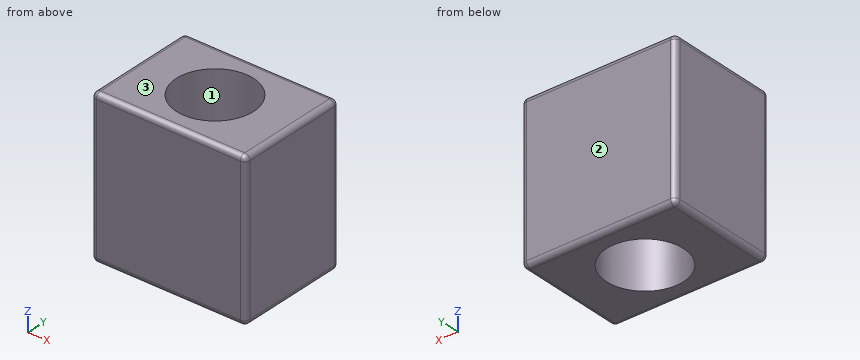
from build123d import *

# Parameters (mm, degrees)
SKETCH1_W           = 15
SKETCH1_H           = 11
SKETCH1_R           = 3.75
BOSS_EXTRUDE1_DEPTH = 7.5
FILLET1_R           = 0.5


with BuildPart() as part:
    # Sketch1 → Boss-Extrude1 (new, symmetric)
    with BuildSketch(Plane.XY):
        Rectangle(SKETCH1_W, SKETCH1_H)
        Circle(SKETCH1_R, mode=Mode.SUBTRACT)
    extrude(amount=BOSS_EXTRUDE1_DEPTH, both=True)

    # Fillet1
    fillet1_edges = [part.edges().sort_by_distance(p)[0] for p in [
        (7.5, 0, 7.5),
        (0, 5.5, 7.5),
        (-7.5, 0, 7.5),
        (0, 5.5, -7.5),
        (7.5, 0, -7.5),
        (0, -5.5, -7.5),
        (-7.5, 0, -7.5),
        (0, -5.5, 7.5),
        (-7.5, 5.5, 0),
        (7.5, 5.5, 0),
        (7.5, -5.5, 0),
        (-7.5, -5.5, 0),
    ]]
    fillet(fillet1_edges, radius=FILLET1_R)


solid = part.part
Read the model definition and answer for the solid it produces. Units are mm, in the model's axes. Face numbers are marked on the shaded views. Round coordinates to 2 decimals unless told otherwise and drop trailing zeros. Write each loop counter-clockwise with the first axis right and the second up, starting at its lowest first coordinate (ties: lowest second). Pieces come first, ordered by that corner, then holes. Notation, with made-up numbers: (13.5, -30) - (43.5, -30) arc R6 ccw to (43.5, -25) - close; hole circle Ø1 at (-20.5, 68.5). An arc over 180 degrees is marked (long way). Use a Markdown table: item, result.
(1) The part is cut by section C-C (y = 0). Write down the section's boundary in (x, z), then the cut area to 3 significant figures.
Reported:
| item | result |
|---|---|
| outline | (-7.5, -7) arc R0.5 ccw to (-7, -7.5) - (-3.75, -7.5) - (-3.75, 7.5) - (-7, 7.5) arc R0.5 ccw to (-7.5, 7) - close; (3.75, -7.5) - (7, -7.5) arc R0.5 ccw to (7.5, -7) - (7.5, 7) arc R0.5 ccw to (7, 7.5) - (3.75, 7.5) - close |
| area | 112 mm2 |
(2) This flat-tipped pin is pushed along its axis until it touches: pin 1 Ø1.5 at (x, y) = (-1.5, -0.5) entering from -Z. Where does it stop, or does it pass through?
Reported:
| item | result |
|---|---|
| pin 1 | through |
(3) The part is cut by section A-A (z = -2.5). Write down the section's boundary in (x, y), then the cut area to 3 significant figures.
Reported:
| item | result |
|---|---|
| outline | (-7.5, -5) arc R0.5 ccw to (-7, -5.5) - (7, -5.5) arc R0.5 ccw to (7.5, -5) - (7.5, 5) arc R0.5 ccw to (7, 5.5) - (-7, 5.5) arc R0.5 ccw to (-7.5, 5) - close; hole circle Ø7.5 at (0, 0) |
| area | 121 mm2 |
(4) Straight lines are drawn through the part: line 1 along Y through (x, z) = (0, 0.75); line 2 along Y through (x, z) = (2.75, -4.5); line 3 along X through (y, z) = (-0.25, 1). For each, find the intervals that lie inside material, in ascending order. Write a range as [from, to].
Reported:
| item | result |
|---|---|
| line 1 | [-5.5, -3.75], [3.75, 5.5] |
| line 2 | [-5.5, -2.55], [2.55, 5.5] |
| line 3 | [-7.5, -3.74], [3.74, 7.5] |
(5) The mould has two halves that part along Y. Classify the marked faces 1, 2 and 3: released by +Y, released by -Y, zero draft, split by the parting line, or undercut.
Reported:
| item | result |
|---|---|
| face 1 | undercut |
| face 2 | released by +Y |
| face 3 | zero draft |
(6) The part is cut by section B-B (x = 0). Write down the section's boundary in (y, z), then the cut area to 3 significant figures.
Reported:
| item | result |
|---|---|
| outline | (-5.5, -7) arc R0.5 ccw to (-5, -7.5) - (-3.75, -7.5) - (-3.75, 7.5) - (-5, 7.5) arc R0.5 ccw to (-5.5, 7) - close; (3.75, -7.5) - (5, -7.5) arc R0.5 ccw to (5.5, -7) - (5.5, 7) arc R0.5 ccw to (5, 7.5) - (3.75, 7.5) - close |
| area | 52.3 mm2 |
